from build123d import *

# Parameters (mm, degrees)
BOSS_EXTRUDE1_DEPTH    = 23
CUT_EXTRUDE1_START     = -12
CUT_EXTRUDE1_DEPTH     = 12
SKETCH4_R              = 17
CUT_EXTRUDE2_DEPTH     = 46
M12X1_5_TAPPED_HOLE1_D = 10.5


# Read off the part's stored shape, not the designer's step: Cut-Extrude1
with BuildPart() as part:
    # Sketch1 → Boss-Extrude1 (new, symmetric)
    with BuildSketch(Plane.XY):
        with BuildLine():
            Line((56, 0), (56, 12))
            Line((56, 12), (31.749015733, 12))
            ThreePointArc((31.749015733, 12), (0, 24), (-31.749015733, 12))
            Line((-31.749015733, 12), (-56, 12))
            Line((-56, 12), (-56, 0))
            Line((-56, 0), (-28, 0))
            Line((-28, 0), (-28, -16))
            Line((-28, -16), (-22.627416998, -16))
            ThreePointArc((-22.627416998, -16), (0, 0), (22.627416998, -16))
            Line((22.627416998, -16), (28, -16))
            Line((28, -16), (28, 0))
            Line((28, 0), (56, 0))
        make_face()
    extrude(amount=BOSS_EXTRUDE1_DEPTH, both=True)

    # Cut-Extrude1 outline → Cut-Extrude1 (cut)
    with BuildSketch(Plane(origin=(0, 12, 0), x_dir=(1, 0, 0), z_dir=(0, 1, 0)).offset(CUT_EXTRUDE1_START)):
        with BuildLine():
            ThreePointArc((-56, 0), (-54.750763557, 11.762393036), (-51.058789645, 23))
            Line((-51.058789645, 23), (-56, 23))
            Line((-56, 23), (-56, 0))
        make_face()
        with BuildLine():
            ThreePointArc((-51.058789645, -23), (-54.750763557, -11.762393036), (-56, 0))
            Line((-56, 0), (-56, -23))
            Line((-56, -23), (-51.058789645, -23))
        make_face()
        with BuildLine():
            Line((56, 23), (51.058789645, 23))
            ThreePointArc((51.058789645, 23), (54.750763557, 11.762393036), (56, 0))
            Line((56, 0), (56, 23))
        make_face()
        with BuildLine():
            Line((56, -23), (56, 0))
            ThreePointArc((56, 0), (54.750763557, -11.762393036), (51.058789645, -23))
            Line((51.058789645, -23), (56, -23))
        make_face()
    extrude(amount=CUT_EXTRUDE1_DEPTH, mode=Mode.SUBTRACT)

    # Sketch4 → Cut-Extrude2 (cut)
    with BuildSketch(Plane(origin=(0, 12, 0), x_dir=(1, 0, 0), z_dir=(0, 1, 0))):
        with Locations((39, 0)):
            Circle(SKETCH4_R)
        with Locations((-39, 0)):
            Circle(SKETCH4_R)
    extrude(amount=CUT_EXTRUDE2_DEPTH, mode=Mode.SUBTRACT)

    # M12x1.5 Tapped Hole1 (through all)
    with Locations(Plane(origin=(39, 12, 0), x_dir=(1, 0, 0), z_dir=(0, 1, 0))):
        with Locations((0, 0)):
            m12x1_5_tapped_hole1 = Hole(M12X1_5_TAPPED_HOLE1_D / 2)

    # Mirror1: M12x1.5 Tapped Hole1 across plane
    add(m12x1_5_tapped_hole1.mirror(Plane(origin=(0, 0, 0), x_dir=(0, 0, 1), z_dir=(1, 0, 0))), mode=Mode.SUBTRACT)

    # Sketch7 → Cut-Revolve4 (revolve, cut)
    with BuildSketch(Plane.XY, mode=Mode.PRIVATE) as cut_revolve4_sk:
        Polygon((0, 24), (4, 24), (4, 8), (3, 8), (3, -2.439893383), (0, -2.439893383), align=None)
    revolve(cut_revolve4_sk.sketch.rotate(Axis((0, 0, 0), (0, 1, 0)), 90), axis=Axis((0, 0, 0), (0, 1, 0)), mode=Mode.SUBTRACT)


solid = part.part
Could you check a few things on this model? Use its own coordinates, in mm. A direction names the side the tool comes from. Coordinates: 2 decimals unless noted, no trailing zeros. Order: outer loops, then holes, each group sorted by start corner. A loop starts at its lowest first (then second) coordinate and runs counter-clockwise, first axis right, second up. Notation, with made-up numbers: (-14, 71) - (1, 71) arc R10 cw to (1, 80) - close; hole circle Ø1 at (-24, 48). An arc over 180 degrees is marked (long way). Answer in a Markdown table with one row per item. Add a question column.
(1) If we section it at C-C, the plane z = 20: Please give me the cut outline in (x, y).
(2) If we mould it in two halves opening along Z, with no side actions, what happens to faces 1 (the face through (-25, -16, 0)), 2 (the face through (22, 15, 0)), 3 (the face through (-1, 9, 23))? For each: released by +Z, released by -Z, zero draft, split by the parting line, or undercut.
(3) On a 3-axis mill with a long thin cutter (end or side, diameter ignored), from which of +Z, -Z, +X, -X, +Y, -Y can I reach the whole of each face in a straight line? I mean faces 4 (the face through (45, 0, 0)), 5 (the face through (43, 12, -5)), 6 (the face through (-43, 12, -5)), 7 (the face through (-28, -8, 0)), 8 (the face through (-3, 8, -1)). Say none if no direction works.
(4) Will these pins go through, and if not, where does the flat tip stop? pin 1 (8.5 mm diameter, centred on x = -38.5, z = 2.5, fed in from -Y); pin 2 (10 mm diameter, centred on x = -41.5, z = -13, fed in from +Y); pin 3 (2 mm diameter, centred on x = -15, z = 17, fed in from +Y).
(5) I need wall thicknesses on L1, parallel to X at y = 13, z = 0; L2, parallel to Z at x = 39, y = 6; L3, parallel to X at y = -12, z = 12. Which ranges of each line are inside material? Lowest first, please.
(6) If we section it at B-B, the plane y = -11.5: Please give me the cut outline in (x, z), then the cut area to 3 significant figures.
(7) If we section it at A-A, the plane x = 0: Please give me the cut outline in (y, z), then the cut area to 3 significant figures.
(8) If we section it at D-D, the plane x = 39: Please give me the cut outline in (y, z).
Results are:
| question | item | result |
|---|---|---|
| 1 | outline | (-52.31, 0) - (-28, 0) - (-28, -16) - (-22.63, -16) arc R24 cw to (22.63, -16) - (28, -16) - (28, 0) - (52.31, 0) - (52.31, 12) - (31.75, 12) arc R48 ccw to (-31.75, 12) - (-52.31, 12) - close |
| 2 | face 1 | zero draft |
| 2 | face 2 | undercut |
| 2 | face 3 | released by +Z |
| 3 | face 4 | +Z, -Z, +X, -Y |
| 3 | face 5 | +X, +Y |
| 3 | face 6 | -X, +Y |
| 3 | face 7 | +Z, -Z, -X, -Y |
| 3 | face 8 | +Y |
| 4 | pin 1 | stops at y = 0 |
| 4 | pin 2 | stops at y = 12 |
| 4 | pin 3 | stops at y = 21.91 |
| 5 | L1 | x = -22 to -4, 4 to 22 |
| 5 | L2 | z = -23 to -5.25, 5.25 to 23 |
| 5 | L3 | x = -28 to -20.78, 20.78 to 28 |
| 6 | outline | (-28, -23) - (-20.49, -23) - (-20.49, 23) - (-28, 23) - close; (20.49, -23) - (28, -23) - (28, 23) - (20.49, 23) - close |
| 6 | area | 691 mm2 |
| 7 | outline | (0, -23) - (24, -23) - (24, -4) - (8, -4) - (8, -3) - (0, -3) - close; (0, 3) - (8, 3) - (8, 4) - (24, 4) - (24, 23) - (0, 23) - close |
| 7 | area | 928 mm2 |
| 8 | outline | (0, -23) - (12, -23) - (12, -5.25) - (0, -5.25) - close; (0, 5.25) - (12, 5.25) - (12, 23) - (0, 23) - close |
